The drawing under review shows one solid part. Ordinate dimensions are in mm from its lowest x, y, z. Coordinates: 2 decimals unless noted, no trailing zeros. Order: outer loops, then holes, each group sorted by start corner. A loop starts at its lowest first (then second) coordinate and runs counter-clockwise, first axis right, second up. Notation, with made-up numbers: (-35, -28.5) -> (11, -28.5) arc R13 ccw to (11, -9.5) -> close; hole circle Ø4 at (-6, 22). An arc over 180 degrees is marked (long way). Write item = value, one per line.
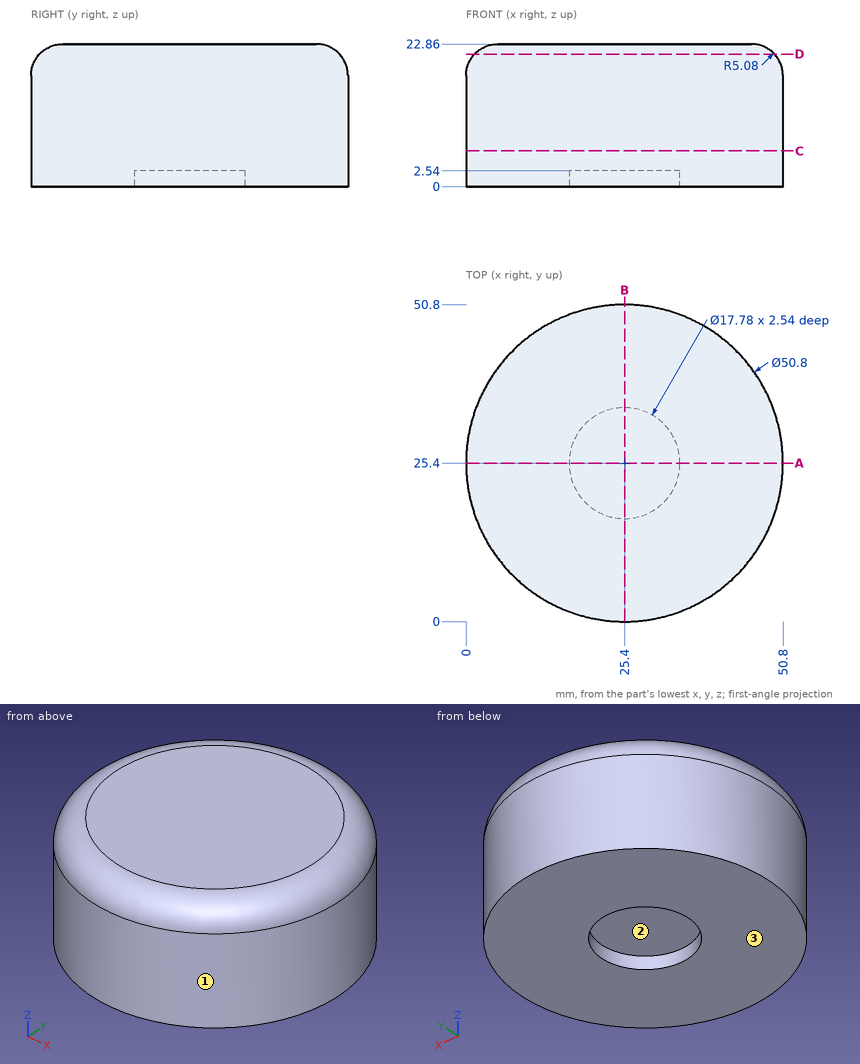
(1) We need section A-A (y = 25.4). Write out the cut boundary in (x, z), and give its area (3 significant figures).
Report:
outline = (0, 0) -> (16.51, 0) -> (16.51, 2.54) -> (34.29, 2.54) -> (34.29, 0) -> (50.8, 0) -> (50.8, 17.78) arc R5.08 ccw to (45.72, 22.86) -> (5.08, 22.86) arc R5.08 ccw to (0, 17.78) -> close
area = 1,110 mm²
(2) Insertion check: pin 1 (9 mm diameter, centred on x = 21, y = 28, fed in from -Z); pin 2 (1.5 mm diameter, centred on y = 43, z = 17, fed in from -X); pin 3 (4 mm diameter, centred on x = 6.5, y = 8.5, fed in from +Z); pin 4 (5 mm diameter, centred on x = 12.5, z = 16.5, fed in from -Y). Each pin has a flat end and moves straight along its axis. Give the tip position at first contact, or say it passes through.
Report:
pin_1 = 0
pin_2 = 6.39
pin_3 = 21.85
pin_4 = 2.23
(3) For L1, parallel to Y at x = 25.4, z = 1.2; L2, parallel to Z at x = 32.5, y = 24.5; L3, parallel to Y at x = 19.5, z = 20.25, list the stretches that pass through material, from the lowest coordinate up.
Report:
L1 = 0 to 16.51, 34.29 to 50.8
L2 = 2.54 to 22.86
L3 = 1.35 to 49.45
(4) The part is to be moulded in two halves that separate along X. For the marked faces 1, 2 and 3, say which applies: released by +X, released by -X, zero draft, split by the parting line, or undercut.
Report:
face_1 = split by the parting line
face_2 = undercut
face_3 = zero draft
(5) We need section D-D (z = 21.25). Write out the cut boundary in (x, y).
Report:
outline = circle Ø48.06 at (25.4, 25.4)
(6) We need section C-C (z = 5.75). Write out the cut boundary in (x, y), and give its area (3 significant figures).
Report:
outline = circle Ø50.8 at (25.4, 25.4)
area = 2,030 mm²
